Source: CAD feature listing. Evaluate the final solid. Frame: model axes, mm. A direction names the side the tool comes from. Give positions to 0.01 mm unless a question says otherwise; leave off trailing zeros. Order: outer loops, then holes, each group sorted by start corner. A loop starts at its lowest first (then second) coordinate and runs counter-clockwise, first axis right, second up.
from build123d import *

# Parameters (mm, degrees)
F0_R     = 46.99
F1_DEPTH = 63.5
F2_W     = 8.8553838432
F2_H     = 43.2049967349
F4_W     = 5.4503902793
F4_H     = 1.6409792006
F4_H_2   = 1.6995854676
F4_H_3   = 2.6958957314
F6_R     = 40.9492493689
F7_DEPTH = 53.975
F8_R     = 11.0109
F9_DEPTH = 50.8


with BuildPart() as f1:
    # F0 (on Top) → F1 (new body)
    with BuildSketch(Plane.XY):
        Circle(F0_R)
    extrude(amount=F1_DEPTH)

    # F2 (on Right) → F3 (revolve, cut)
    with BuildSketch(Plane.YZ):
        with Locations((-48.5519412905, 21.6024983674)):
            Rectangle(F2_W, F2_H)
    revolve(axis=Axis((0, 0, 0), (0, 0, 1)), mode=Mode.SUBTRACT)

    # F4 (on Right) → F5 (revolve, cut)
    with BuildSketch(Plane.YZ):
        with Locations((-46.1188144982, 53.4723494202)):
            Rectangle(F4_W, F4_H)
        with Locations((-46.1188144982, 50.6885442883)):
            Rectangle(F4_W, F4_H_2)
        with Locations((-46.1188144982, 46.9670407474)):
            Rectangle(F4_W, F4_H_3)
    revolve(axis=Axis((0, 0, 43.2049967349), (0, 0, -1)), mode=Mode.SUBTRACT)

    # F6 (on face) → F7 (cut)
    with BuildSketch(Plane(origin=(0, 0, 0), x_dir=(1, 0, 0), z_dir=(0, 0, -1))):
        Circle(F6_R)
    extrude(amount=-F7_DEPTH, mode=Mode.SUBTRACT)

    # F8 (on Right) → F9 (cut, symmetric)
    with BuildSketch(Plane.YZ):
        with BuildLine():
            add(Edge.make_bspline(
                [(-46.9745136797, 31.0811214149), (-40.0877244728, 27.5083131565), (-27.2735309688, 20.8604174535), (-16.9769809248, 7.2973682669), (-15.9815300532, -11.6642689281), (-15.8178017222, -17.9375006966), (-15.7510973513, -20.4932708293)],
                knots=[0, 0, 0, 0, 0.2945724143, 0.5481085314, 0.815895417, 1, 1, 1, 1], degree=3))
            Line((-46.9745136797, 31.0811214149), (-50.5986586213, -20.4932708293))
            Line((-50.5986586213, -20.4932708293), (-15.7510973513, -20.4932708293))
        make_face()
        with Locations((0, 16.026975587)):
            Circle(F8_R)
        with BuildLine():
            Line((50.5986586213, -20.4932708293), (46.9745136797, 31.0811214149))
            add(Edge.make_bspline(
                [(46.9745136797, 31.0811214149), (40.0877244728, 27.5083131565), (27.2735309688, 20.8604174535), (16.9769809248, 7.2973682669), (15.9815300532, -11.6642689281), (15.8178017222, -17.9375006966), (15.7510973513, -20.4932708293)],
                knots=[0, 0, 0, 0, 0.2945724143, 0.5481085314, 0.815895417, 1, 1, 1, 1], degree=3))
            Line((15.7510973513, -20.4932708293), (50.5986586213, -20.4932708293))
        make_face()
    extrude(amount=F9_DEPTH, both=True, mode=Mode.SUBTRACT)


solid = f1.part
(1) Pin query (flat end, axial travel): pin 1 Ø1.5 at (x, z) = (-32.5, 30) entering from +Y; pin 2 Ø12 at (x, z) = (-15.5, 19) entering from +Y; pin 3 Ø10 at (y, z) = (24, 32.5) entering from -X; pin 4 Ø12 at (x, y) = (-18, 8) entering from -Z (3 decimals). Return the tip coordinate at first contact, or that it passes through.
(2) Line query: line 1 along Y through (x, z) = (-37, 10); line 2 along Z through (x, y) = (1, 31) (3 decimals); line 3 along Y through (x, z) = (0, 38). Output: solid intervals per line, ascending.
(3) Draft query along Z for faces 1 (the cylindrical face through (-10.19, -45.87, 58.83)), 2 (the flat face through (-41.5, 0.2, 0)), 3 (the flat face through (14, -42, 54.293)), 4 (the cylindrical face through (26.4, 34.44, 46.99)). Return one class per face: +Z half, -Z half, draft (parallel to the pull), parting line (faces both ways), or undercut.
(4) Access query for faces 5 (the cylindrical face through (-39.146, -20.361, 31.506)), 6 (the cylindrical face through (-10.19, -45.87, 44.4)), 7 (the flat face through (14, -42, 52.652)). Directions: +Z, -Z, +X, -X, +Y, -Y. A direction counts if a zero-diameter tool reaches every point of the face in a straight line with its end or side. Return the directions, or none.
(5) Section A-A, the plane y = 0. Count the separate pieces of the cut face and the enclosed holes in it, plus the area to 3 significant figures.
(6) Section B-B, the plane z = 37.5. Return loops of the section in (x, y), plus the area to 3 significant figures.
Checks:
1. pin 1: stops at y = 30.64
1. pin 2: passes through
1. pin 3: stops at x = -39.82
1. pin 4: stops at z = 53.975
2. line 1: y = -20.08 to -17.55, 17.55 to 20.08
2. line 2: z = 53.975 to 63.5
2. line 3: y = -44.12 to -40.95, 40.95 to 44.12
3. face 1: draft
3. face 2: -Z half
3. face 3: undercut
3. face 4: undercut
4. face 5: -Z
4. face 6: +Z, -Z
4. face 7: none
5. separate pieces: 3
5. enclosed holes: 0
5. area: 1,120 mm2
6. outline: circle Ø88.25 at (0, 0); hole circle Ø81.9 at (0, 0)
6. area: 849 mm2
